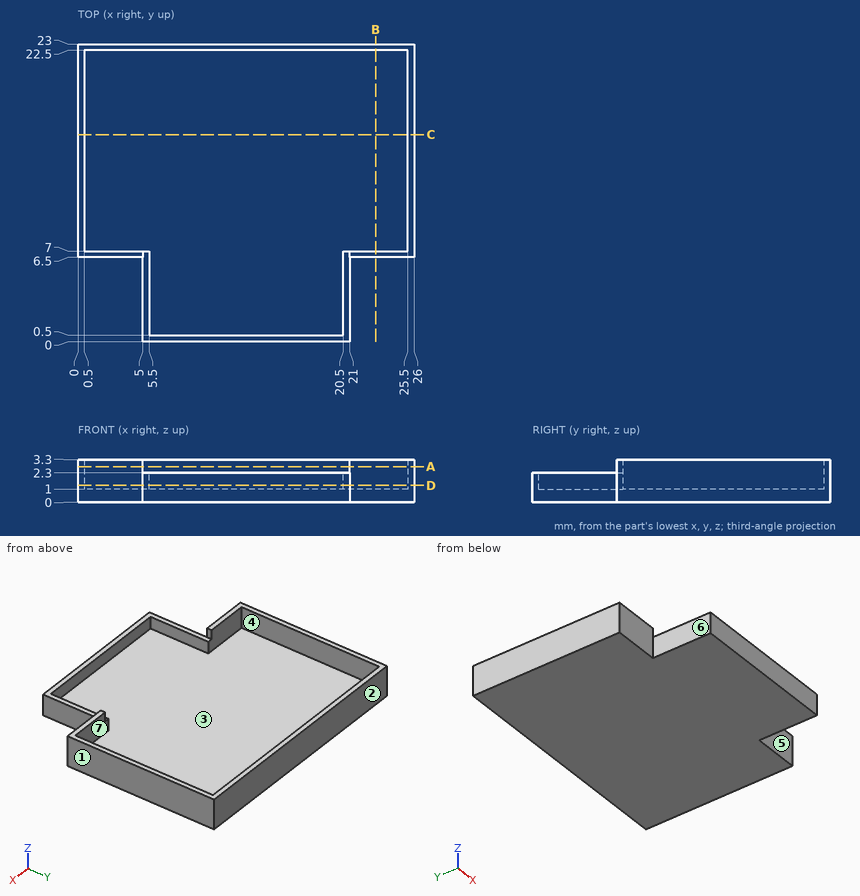
Study the drawing (mm; zero at the part's minimum x, y, z) and answer. A direction names the side the tool comes from. Coordinates: 2 decimals unless noted, no trailing zeros. Write each loop counter-clockwise with the first axis right and the second up, starting at its lowest first coordinate (ties: lowest second). Pieces come first, ordered by that corner, then holes.
Q1. A cutting plane is placed at D-D, the plane z = 1.3. Give the vertices of the cut face in (x, y), then the cut area to 3 significant figures.
Q2. Find the intervals of material crossed by line 1 (Y direction, x = 2.25, z = 1.2); line 2 (X direction, y = 8.75, z = 2.25); line 3 (Y direction, x = 13, z = 1.35), in increasing order.
Q3. Each of these flat-tipped pins is pushed along its axis until it touches: pin 1 Ø1 at (x, z) = (23, 1) entering from -Y; pin 2 Ø0.7 at (y, z) = (2, 1.5) entering from +X; pin 3 Ø2 at (x, y) = (16.5, 4.5) entering from +Z. Where does it stop, or does it pass through?
Q4. A cutting plane is placed at A-A, the plane z = 2.75. Give the vertices of the cut face in (x, y), then the cut area to 3 significant figures.
Q5. Which of the six approach directions +Z, -Z, +X, -X, +Y, -Y give full straight-line access (tool end or side, diameter ignored) to the marked faces 5, 6 and 7?
Q6. Determine the mould class of the marked faces 1, 2, 3 and 4 for opening direction X: released by +X, released by -X, zero draft, split by the parting line, or undercut.
Q7. A cutting plane is placed at C-C, the plane y = 16. Give the vertices of the cut face in (x, z), then the cut area to 3 significant figures.
Q8. A cutting plane is placed at B-B, the plane x = 23. Give the vertices of the cut face in (y, z), then the cut area to 3 significant figures.
Findings below:
1. outline: (0, 6.5) - (5, 6.5) - (5, 0) - (21, 0) - (21, 6.5) - (26, 6.5) - (26, 23) - (0, 23) - close; hole (0.5, 7) - (5.5, 7) - (5.5, 0.5) - (20.5, 0.5) - (20.5, 7) - (25.5, 7) - (25.5, 22.5) - (0.5, 22.5) - close
1. area: 48.0 mm2
2. line 1: y = 6.5 to 7, 22.5 to 23
2. line 2: x = 0 to 0.5, 25.5 to 26
2. line 3: y = 0 to 0.5, 22.5 to 23
3. pin 1: stops at y = 6.5
3. pin 2: stops at x = 21
3. pin 3: stops at z = 1
4. outline: (0, 6.5) - (5, 6.5) - (5, 7) - (0.5, 7) - (0.5, 22.5) - (25.5, 22.5) - (25.5, 7) - (21, 7) - (21, 6.5) - (26, 6.5) - (26, 23) - (0, 23) - close
4. area: 33.5 mm2
5. face 5: +Z, -Z, +X, -Y
5. face 6: +Z, -Z, -X, -Y
5. face 7: +Z
6. face 1: released by +X
6. face 2: zero draft
6. face 3: undercut
6. face 4: undercut
7. outline: (0, 0) - (26, 0) - (26, 3.3) - (25.5, 3.3) - (25.5, 1) - (0.5, 1) - (0.5, 3.3) - (0, 3.3) - close
7. area: 28.3 mm2
8. outline: (6.5, 0) - (23, 0) - (23, 3.3) - (22.5, 3.3) - (22.5, 1) - (7, 1) - (7, 3.3) - (6.5, 3.3) - close
8. area: 18.8 mm2
